The figure shows three views and two pictorial views of one solid part (mm, origin at its lowest corner). Answer the questions. A direction names the side the tool comes from. Give positions to 0.01 mm unless a question says otherwise; leave off trailing zeros. Order: outer loops, then holes, each group sorted by start corner. A loop starts at its lowest first (then second) coordinate and runs counter-clockwise, first axis right, second up. Notation, with made-up numbers: (74.5, 4) - (88.5, 4) arc R20 cw to (88.5, 19) - close; hole circle Ø7 at (-1.75, -6.5). An arc over 180 degrees is marked (long way). Answer as a JSON object with one key per item and string values. Group by question number.
Q1. A cutting plane is placed at B-B, the plane y = 45. Give the vertices of the cut face in (x, z), and give its area (3 significant figures).
Q2. For the marked faces 1, 2 and 3, determine the directions among +Z, -Z, +X, -X, +Y, -Y from which every point of the face is accessible in a straight line to the end or side of a thin tool.
Q3. A cutting plane is placed at A-A, the plane z = 45. Give the vertices of the cut face in (x, y).
Q4. Consider line 1 (X direction, y = 67, z = 14); line 2 (Z direction, x = 80.5, y = 37.5); line 3 (Z direction, x = 27.5, y = 67). Determine where each line is inside the solid, lowest interval first.
Q5. Given pin 1 (1 mm diameter, centred on y = 56, z = 16, fed in from -X); pin 2 (5 mm diameter, centred on x = 74.5, y = 39, fed in from +Z); pin 3 (6 mm diameter, centred on x = 77, y = 26.5, fed in from +Z); pin 4 (12 mm diameter, centred on x = 67.5, z = 42.5, fed in from +Y), each flat-ended and moving along its own axis, determine where each tip first touches the part or whether it passes through.
Q6. A cutting plane is placed at C-C, the plane x = 58. Give the vertices of the cut face in (y, z), and give its area (3 significant figures).
Q7. A cutting plane is placed at D-D, the plane y = 76.06. Give the vertices of the cut face in (x, z).
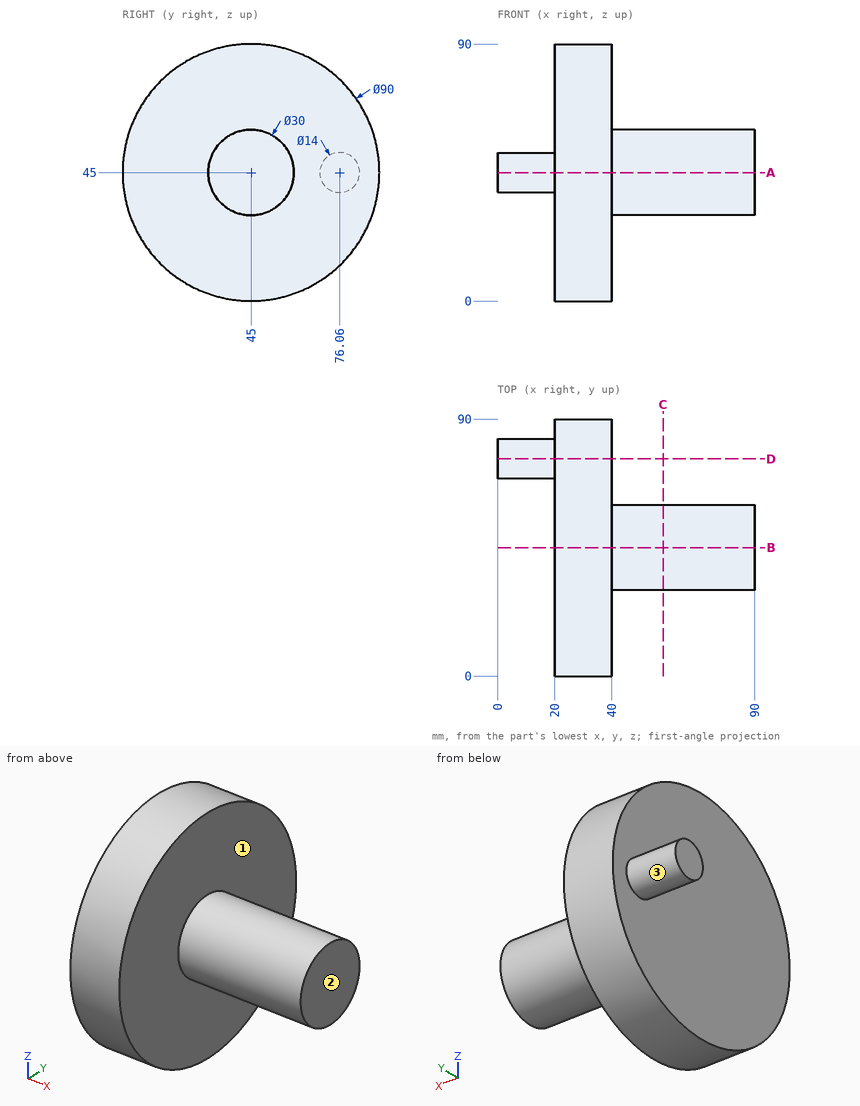
Reply:
{
 "1": {"outline": "(20, 0) - (40, 0) - (40, 30) - (90, 30) - (90, 60) - (40, 60) - (40, 90) - (20, 90) - close", "area": "3,300 mm^2"},
 "2": {"face 1": "+X", "face 2": "+Z, -Z, +X, +Y, -Y", "face 3": "-X"},
 "3": {"outline": "(0, 69.06) - (20, 69.06) - (20, 0) - (40, 0) - (40, 30) - (90, 30) - (90, 60) - (40, 60) - (40, 90) - (20, 90) - (20, 83.06) - (0, 83.06) - close"},
 "4": {"line 1": "x = 20 to 40", "line 2": "z = 32.01 to 57.99", "line 3": "z = 5.74 to 84.26"},
 "5": {"pin 1": "stops at x = 20", "pin 2": "stops at z = 59.59", "pin 3": "passes through", "pin 4": "stops at y = 60"},
 "6": {"outline": "circle Ø30 at (45, 45)", "area": "707 mm^2"},
 "7": {"outline": "(0, 38) - (20, 38) - (20, 12.44) - (40, 12.44) - (40, 77.56) - (20, 77.56) - (20, 52) - (0, 52) - close"}
}
